```python
from build123d import *

# Parameters (mm, degrees)
EXTRUDE_1_DEPTH     = 4
SKETCH_4_R          = 17.5
EXTRUDE_2_DEPTH     = 8
SKETCH_3_R          = 11
CUT_EXTRUDE_1_DEPTH = 7
FILLET_5_R          = 7.5
FILLET_6_R          = 10
FILLET_7_R          = 8
SKETCH_5_R          = 4
CUT_EXTRUDE_2_DEPTH = 71.900963896
SKETCH_6_R          = 6.25
CUT_EXTRUDE_3_DEPTH = 0.4


with BuildPart() as part:
    # 草圖1 → 填料-伸長1 (new body)
    with BuildSketch(Plane(origin=(0, 0, 0), x_dir=(1, 0, 0), z_dir=(0, 1, 0))):
        with BuildLine():
            Line((-24, -7.5), (-12.990381057, -7.5))
            ThreePointArc((-12.990381057, -7.5), (-14.488887394, -3.882285677), (-15, 0))
            Line((-15, 0), (-24, 0))
            Line((-24, 0), (-24, -7.5))
        make_face()
        with BuildLine():
            ThreePointArc((-15, 0), (-14.488887394, 3.882285677), (-12.990381057, 7.5))
            Line((-12.990381057, 7.5), (-24, 7.5))
            Line((-24, 7.5), (-24, 0))
            Line((-24, 0), (-15, 0))
        make_face()
        with BuildLine():
            ThreePointArc((-4, 0), (0, 4), (4, 0))
            Line((4, 0), (15, 0))
            ThreePointArc((15, 0), (3.882285677, 14.488887394), (-12.990381057, 7.5))
            ThreePointArc((-12.990381057, 7.5), (-14.488887394, 3.882285677), (-15, 0))
            Line((-15, 0), (-4, 0))
        make_face()
        with BuildLine():
            Line((15, 0), (4, 0))
            ThreePointArc((4, 0), (0, -4), (-4, 0))
            Line((-4, 0), (-15, 0))
            ThreePointArc((-15, 0), (-14.488887394, -3.882285677), (-12.990381057, -7.5))
            ThreePointArc((-12.990381057, -7.5), (3.882285677, -14.488887394), (15, 0))
        make_face()
    extrude(amount=EXTRUDE_1_DEPTH)

    # 草圖4 → 填料-伸長2 (add)
    with BuildSketch(Plane.ZY.offset(24)):
        with Locations((0, 39.742437699)):
            Circle(SKETCH_4_R)
        with BuildLine():
            ThreePointArc((7.5, 23.931049399), (0, 22.242437699), (-7.5, 23.931049399))
            Line((-7.5, 23.931049399), (-7.5, 4))
            Line((-7.5, 4), (7.5, 4))
            Line((7.5, 4), (7.5, 23.931049399))
        make_face()
    extrude(amount=-EXTRUDE_2_DEPTH)

    # 草圖3 → 除料-伸長1 (cut)
    with BuildSketch(Plane.ZY.offset(16)):
        with Locations((0, 40)):
            Circle(SKETCH_3_R)
    extrude(amount=CUT_EXTRUDE_1_DEPTH, mode=Mode.SUBTRACT)

    # 圓角5
    fillet_5_edges = [part.edges().sort_by_distance(p)[0] for p in [
        (-12.990381057, 2, -7.5),
    ]]
    fillet(fillet_5_edges, radius=FILLET_5_R)
    fillet_5_2_edges = [part.edges().sort_by_distance(p)[0] for p in [
        (-12.990381057, 2, 7.5),
    ]]
    fillet(fillet_5_2_edges, radius=FILLET_5_R)

    # 圓角6
    # the kernel refuses this fillet: 10 mm, written as the material it adds along each edge
    with BuildSketch(Plane(origin=(-24, 23.931049399, -7.5), x_dir=(0, -1, 0), z_dir=(1, 0, 0))) as fillet_6_piece_1_section:
        with BuildLine():
            CenterArc((5.401815135, 10), FILLET_6_R, 219.521196359, 50.478803641)
            ThreePointArc((-2.312077024, 3.636363636), (-1.04368494, 1.889618599), (0, 0))
            Line((0, 0), (5.401815135, 0))
        make_face()
    fillet_6_piece_1 = extrude(amount=20.734028006, mode=Mode.PRIVATE)
    fillet_6_piece_1 = split(fillet_6_piece_1, bisect_by=Plane(origin=(-16, 22.860103081, -8.083386196), z_dir=(-1, 0, 0)), keep=Keep.TOP, mode=Mode.PRIVATE)
    add(fillet_6_piece_1)
    with BuildSketch(Plane(origin=(-24, 23.931049399, 7.5), x_dir=(0, -1, 0), z_dir=(1, 0, 0))) as fillet_6_piece_2_section:
        with BuildLine():
            CenterArc((5.401815135, -10), FILLET_6_R, 90, 50.478803641)
            ThreePointArc((-2.312077024, -3.636363636), (-1.04368494, -1.889618599), (0, 0))
            Line((0, 0), (5.401815135, 0))
        make_face()
    fillet_6_piece_2 = extrude(amount=20.734028006, mode=Mode.PRIVATE)
    fillet_6_piece_2 = split(fillet_6_piece_2, bisect_by=Plane(origin=(-16, 22.860102946, 8.083386188), z_dir=(-1, 0, 0)), keep=Keep.TOP, mode=Mode.PRIVATE)
    add(fillet_6_piece_2)

    # 圓角7
    fillet_7_edges = [part.edges().sort_by_distance(p)[0] for p in [
        (-16, 4, 0),
    ]]
    fillet(fillet_7_edges, radius=FILLET_7_R)

    # 草圖5 → 除料-伸長2 (cut, through all)
    with BuildSketch(Plane(origin=(-23, 0, 0), x_dir=(0, 0, -1), z_dir=(1, 0, 0))):
        with Locations((0, 40)):
            Circle(SKETCH_5_R)
    extrude(amount=-CUT_EXTRUDE_2_DEPTH, mode=Mode.SUBTRACT)

    # 草圖6 → 除料-伸長3 (cut)
    with BuildSketch(Plane(origin=(-23, 0, 0), x_dir=(0, 0, -1), z_dir=(1, 0, 0))):
        with Locations((0, 40)):
            Circle(SKETCH_6_R)
    extrude(amount=-CUT_EXTRUDE_3_DEPTH, mode=Mode.SUBTRACT)


solid = part.part
```
Can you work these out from the model? Positions are in its coordinate system, mm. A direction names the side the tool comes from. Round coordinates to 2 decimals unless told otherwise and drop trailing zeros. Loops run counter-clockwise (first coordinate to the right, second up) from the corner with the lowest first, then second, coordinate; pieces in that order, holes last.
Item 1: Suppose I cut it at D-D, the plane x = -20.5. Write out the boundary of the cut face in (y, z), then the cut area to 3 significant figures.
Item 2: Suppose I cut it at A-A, the plane x = 0. Write out the boundary of the cut face in (y, z).
Item 3: If we mould it in two halves opening along Z, with no side actions, what happens to faces 1 (the cylindrical face through (-20.06, 22.85, -8.48)), 2 (the cylindrical face through (-14.403, 5.53, 7.884)), 3 (the cylindrical face through (-0.867, 1.972, -3.905))? For each: +Z half, -Z half, draft (parallel to the pull), parting line (faces both ways), or undercut.
Item 4: Please list where these lines run through material, in increasing order: L1, parallel to X at y = 13, z = -6; L2, parallel to Y at x = -1, z = 7.5; L3, parallel to X at y = 46, z = 1.5.
Item 5: Suppose I cut it at B-B, the plane y = 41. Write out the boundary of the cut face in (x, z), then the cut area to 3 significant figures.
Item 6: Suppose I cut it at C-C, the plane z = -13.5. Write out the boundary of the cut face in (x, y), then the cut area to 3 significant figures.
Item 7: Will these pins go through, and if not, where does the flat tip stop? pin 1 Ø17.5 at (y, z) = (35, -2) entering from +X; pin 2 Ø7.5 at (y, z) = (40, 0) entering from +X; pin 3 Ø1.5 at (x, z) = (-15, -5.5) entering from -Y; pin 4 Ø2 at (x, y) = (-19, 14) entering from +Z.
Item 8: Which directions (+Z, -Z, +X, -X, +Y, -Y) give clear straight access to the entire face, cutting with the end or side of a thin tool? Please do faces 4 (the flat face through (-20, 9, -7.5)), 5 (the flat face through (-23, 35, 5)), 6 (the flat face through (3, 4, 3)).
Reported:
1. outline: (0, -7.5) - (18.53, -7.5) arc R10 cw to (26.24, -11.14) arc R17.5 ccw (long way) to (26.24, 11.14) arc R10 cw to (18.53, 7.5) - (0, 7.5) - close; hole circle Ø22 at (40, 0)
1. area: 932 mm2
2. outline: (0, -15) - (4, -15) - (4, -4) - (0, -4) - close; (0, 4) - (4, 4) - (4, 15) - (0, 15) - close
3. face 1: -Z half
3. face 2: +Z half
3. face 3: undercut
4. L1: x = -24 to -16
4. L2: y = 0 to 4
4. L3: x = -24 to -23.4
5. outline: (-24, -17.45) - (-16, -17.45) - (-16, -10.95) - (-23, -10.95) - (-23, -6.17) - (-23.4, -6.17) - (-23.4, -3.87) - (-24, -3.87) - close; (-24, 3.87) - (-23.4, 3.87) - (-23.4, 6.17) - (-23, 6.17) - (-23, 10.95) - (-16, 10.95) - (-16, 17.45) - (-24, 17.45) - close
5. area: 116 mm2
6. outline: (-24, 28.61) - (-16, 28.61) - (-16, 50.88) - (-24, 50.88) - close; (-6.54, 0) - (6.54, 0) - (6.54, 4) - (-6.54, 4) - close
6. area: 230 mm2
7. pin 1: stops at x = -16
7. pin 2: passes through
7. pin 3: stops at y = 0
7. pin 4: stops at z = 7.5
8. face 4: -Z, -X, -Y
8. face 5: +X
8. face 6: +Z, -Z, +X, +Y
